from build123d import *

# Parameters (mm, degrees)
BOSS_EXTRUDE1_DEPTH = 25
FILLET1_R           = 0.5
FILLET2_R           = 0.5
BOSS_EXTRUDE2_DEPTH = 25


with BuildPart() as part:
    # Sketch6 → Boss-Extrude1 (new body)
    with BuildSketch(Plane(origin=(0, 0, 0), x_dir=(1, 0, 0), z_dir=(0, 1, 0))):
        with BuildLine():
            Line((-23.5, 1.5), (-4, 1.5))
            Line((-4, 1.5), (-4, 8.5))
            Line((-4, 8.5), (-6, 8.5))
            Line((-6, 8.5), (-6, 10))
            Line((-6, 10), (-2.5, 10))
            Line((-2.5, 10), (-2.5, 6))
            ThreePointArc((-2.5, 6), (-1.840169944, 3.204915028), (0, 1))
            ThreePointArc((0, 1), (1.840169944, 3.204915028), (2.5, 6))
            Line((2.5, 6), (2.5, 10))
            Line((2.5, 10), (6, 10))
            Line((6, 10), (6, 8.5))
            Line((6, 8.5), (4, 8.5))
            Line((4, 8.5), (4, 1.5))
            Line((4, 1.5), (23.5, 1.5))
            Line((23.5, 1.5), (23.5, 2))
            Line((23.5, 2), (23, 3))
            Line((23, 3), (25, 3))
            Line((25, 3), (25, 0))
            Line((25, 0), (2.5, 0))
            Line((2.5, 0), (-2.5, 0))
            Line((-2.5, 0), (-25, 0))
            Line((-25, 0), (-25, 3))
            Line((-25, 3), (-23, 3))
            Line((-23, 3), (-23.5, 2))
            Line((-23.5, 2), (-23.5, 1.5))
        make_face()
    extrude(amount=BOSS_EXTRUDE1_DEPTH)

    # Fillet1
    fillet1_edges = [part.edges().sort_by_distance(p)[0] for p in [
        (-4, 12.5, -1.5),
        (-4, 12.5, -8.5),
        (0, 12.5, -1),
        (4, 12.5, -8.5),
        (4, 12.5, -1.5),
    ]]
    fillet(fillet1_edges, radius=FILLET1_R)

    # Fillet2
    fillet2_edges = [part.edges().sort_by_distance(p)[0] for p in [
        (-6, 12.5, -8.5),
        (-6, 12.5, -10),
        (-2.5, 12.5, -10),
        (2.5, 12.5, -10),
        (6, 12.5, -10),
        (6, 12.5, -8.5),
        (25, 12.5, -3),
        (25, 12.5, 0),
        (-25, 12.5, 0),
        (-25, 12.5, -3),
    ]]
    fillet(fillet2_edges, radius=FILLET2_R)

    # Sketch7 → Boss-Extrude2 (add)
    with BuildSketch(Plane(origin=(0, 25, 0), x_dir=(1, 0, 0), z_dir=(0, 1, 0))):
        Polygon((-19.5, 0), (-19.5, -2.75), (-14.5, -2.75), (-16, -1.25), (-17.5, -1.25), (-17.5, 0), align=None)
        Polygon((19.5, 0), (17.5, 0), (17.5, -1.25), (16, -1.25), (14.5, -2.75), (19.5, -2.75), align=None)
    extrude(amount=-BOSS_EXTRUDE2_DEPTH)


solid = part.part
The model under review builds one solid part; all positions refer to its coordinate system, in mm. A direction names the side the tool comes from. Round coordinates to 2 decimals unless told otherwise and drop trailing zeros. Write each loop counter-clockwise with the first axis right and the second up, starting at its lowest first coordinate (ties: lowest second). Pieces come first, ordered by that corner, then holes. Notation, with made-up numbers: (62.5, -11.75) - (121.5, -11.75) arc R8 ccw to (121.5, 1.25) - close; hole circle Ø2 at (24.25, -34.75). An arc over 180 degrees is marked (long way). One line per item, written item: value. Start each with the question number.
1. Consider section A-A on z = 0.75. Write out the cut boundary in (x, y), and give its area (3 significant figures).
2. Clearance check with flat-ended pins moving along their axes: P1, Ø5, axis at x = 9.5, y = 15, coming from the -Z side; P2, Ø1.4, axis at y = 10.5, z = 0.5, coming from the -X side; P3, Ø4, axis at x = 5, y = 6, coming from the +Z side; P4, Ø8, axis at x = 13, y = 6, coming from the +Z side. State where each tip first meets the part, or that it passes through.
3. Consider section B-B on x = 5. Write out the cut boundary in (y, z).
4. Consider section D-D on x = 18. Write out the cut boundary in (y, z).
5. To check wall thickness, follow L1, parallel to Z at x = 5, y = 13.75; L2, parallel to X at y = 22.75, z = -9.25; L3, parallel to X at y = 3.5, z = -8. State the ranges of each line that lie inside material, in increasing order. Write a range as from..to.
6. The part is to be moulded in two halves that separate along Z. For faces 1 (the face through (17, 13, 2.75)), 2 (the face through (2, 0, -2)), 3 (the face through (-17.5, 13, 1)), say which applies: released by +Z, released by -Z, zero draft, split by the parting line, or undercut.
7. Machinability: for faces 4 (the face through (-2.5, 12, -8)), 5 (the face through (-4, 12, -5)), 6 (the face through (24, 12, -3)), 7 (the face through (-19.5, 13, 1)), which of the approach directions +Z, -Z, +X, -X, +Y, -Y give a long, thin tool a straight path to every point of the face, cutting with its end or side? Answer none if there is none.
8. Consider section C-C on x = 11. Write out the cut boundary in (y, z), and give its area (3 significant figures).
Checks:
1. outline: (-19.5, 0) - (-17.5, 0) - (-17.5, 25) - (-19.5, 25) - close; (17.5, 0) - (19.5, 0) - (19.5, 25) - (17.5, 25) - close
1. area: 100 mm^2
2. P1: stops at z = -1.5
2. P2: stops at x = -24.9
2. P3: stops at z = 0
2. P4: stops at z = 2.75
3. outline: (0, -10) - (25, -10) - (25, -8.5) - (0, -8.5) - close; (0, -1.5) - (25, -1.5) - (25, 0) - (0, 0) - close
4. outline: (0, -1.5) - (25, -1.5) - (25, 2.75) - (0, 2.75) - close
5. L1: z = -10..-8.5, -1.5..0
5. L2: x = -6..-2.5, 2.5..6
5. L3: x = -4..-2.5, 2.5..4
6. face 1: released by +Z
6. face 2: zero draft
6. face 3: undercut
7. face 4: -Z, +Y, -Y
7. face 5: +Y, -Y
7. face 6: -Z, +X, +Y, -Y
7. face 7: +Z, -X, +Y, -Y
8. outline: (0, -1.5) - (25, -1.5) - (25, 0) - (0, 0) - close
8. area: 37.5 mm^2
